Could you check a few things on this drawing? It's one solid part, dimensions in mm from its lowest x, y, z. Coordinates: 2 decimals unless noted, no trailing zeros. Write each loop counter-clockwise with the first axis right and the second up, starting at its lowest first coordinate (ties: lowest second). Pieces come first, ordered by that corner, then holes. Notation, with made-up numbers: M 40,-6 L 55,-6 A33 cw 55,27 Z; hole C -34,57.25 d9. An arc over 180 degrees is marked long. Use a Markdown table: item, result.
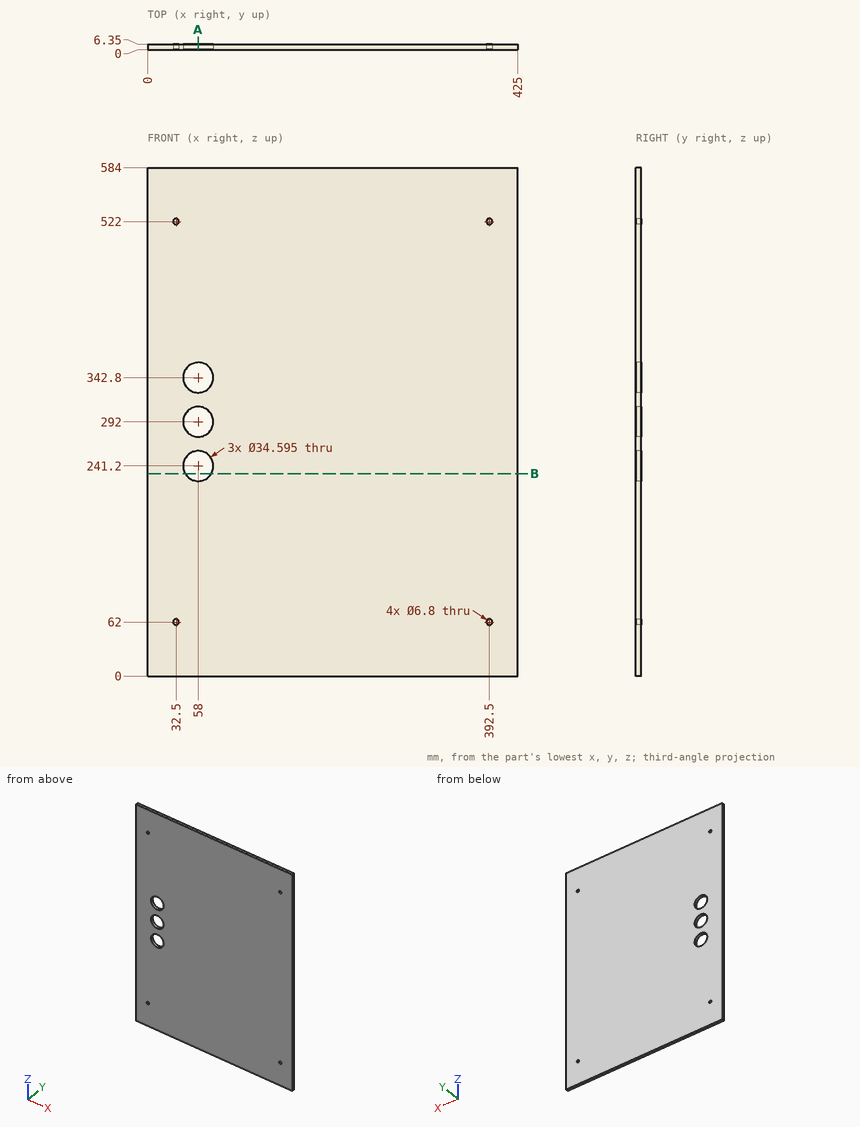
1. Will these pins go through, and if not, where does the flat tip stop? pin 1 Ø21 at (x, z) = (58, 342.8) entering from +Y; pin 2 Ø9 at (x, z) = (32.5, 522) entering from -Y.
Answers follow:
| item | result |
|---|---|
| pin 1 | passes through |
| pin 2 | stops at y = 0 |
2. Suppose I cut it at B-B on z = 232.5. Write out the boundary of the cut face in (x, y).
Answers follow:
| item | result |
|---|---|
| outline | M 0,0 L 43.05,0 L 43.05,6.35 L 0,6.35 Z; M 72.95,0 L 425,0 L 425,6.35 L 72.95,6.35 Z |
3. I need wall thicknesses on probe 1 along Z at (x, y) = (58, 4); probe 2 along Z at (x, y) = (32.5, 3.5); probe 3 along X at (y, z) = (2.5, 62). Which ranges of each line are inside material? Lowest first, please.
Answers follow:
| item | result |
|---|---|
| probe 1 | z = 0 to 223.9, 258.5 to 274.7, 309.3 to 325.5, 360.1 to 584 |
| probe 2 | z = 0 to 58.6, 65.4 to 518.6, 525.4 to 584 |
| probe 3 | x = 0 to 29.1, 35.9 to 389.1, 395.9 to 425 |
4. Suppose I cut it at A-A on x = 58. Write out the boundary of the cut face in (y, z).
Answers follow:
| item | result |
|---|---|
| outline | M 0,0 L 6.35,0 L 6.35,223.9 L 0,223.9 Z; M 0,258.5 L 6.35,258.5 L 6.35,274.7 L 0,274.7 Z; M 0,309.3 L 6.35,309.3 L 6.35,325.5 L 0,325.5 Z; M 0,360.1 L 6.35,360.1 L 6.35,584 L 0,584 Z |
